Input: part model. Units: mm. Frame: model coordinates. A direction names the side the tool comes from. Coordinates: 2 decimals unless noted, no trailing zeros. Loops run counter-clockwise (first coordinate to the right, second up) from the corner with the lowest first, then second, coordinate; pieces in that order, holes last.
(1) Section B-B, the plane y = 36. Return loops of the section in (x, z).
(2) Section A-A, the plane x = 65. Return loops of the section in (y, z), then the cut area to 3 significant figures.
(3) Line query: L1, parallel to Y at x = 65, z = 6.25; L2, parallel to X at y = 36, z = 5; L3, parallel to Z at x = 35.5, y = 26. Output: solid intervals per line, ascending.
(4) Section D-D, the plane y = 20.5. Return loops of the section in (x, z), then the cut area to 3 significant figures.
(5) Contact query for flat-ended pins moving along their axis: P1, Ø1, axis at x = 39, z = 14, coming from the +Y side; P2, Ø1.6, axis at y = 5.5, z = 14.5, coming from the -X side. Output: stop coordinate, or through.
(6) Set-up query: faces 4 (the face through (49, 7, 14)), 5 (the face through (19, 7, 14)), 6 (the face through (34, 14, 14)). Return all of +Z, -Z, +X, -X, +Y, -Y with unobstructed straight access to the full face (end or side cutting, diameter ignored); none if empty.
(7) Mould query, pull axis Y, two halves, no side actions, for faces 1 (the face through (67.4, 0.57, 6.59)), 2 (the face through (3.325, 37.464, 6.409)), 3 (the face through (34, 20, 0)). Classes: released by +Y, released by -Y, zero draft, split by the parting line, or undercut.
(8) Section C-C, the plane x = 32.5. Return loops of the section in (y, z), then the cut area to 3 significant figures.
```python
from build123d import *

# Parameters (mm, degrees)
CROQUIS1_W              = 68
CROQUIS1_H              = 39
CROQUIS1_R              = 1.5
SALIENTE_EXTRUIR1_DEPTH = 13
REDONDEO1_R             = 2
CROQUIS2_W              = 30
CROQUIS2_H              = 14
SALIENTE_EXTRUIR2_DEPTH = 2


with BuildPart() as part:
    # Croquis1 → Saliente-Extruir1 (new body)
    with BuildSketch(Plane.XY):
        with Locations((34, 19.5)):
            Rectangle(CROQUIS1_W, CROQUIS1_H)
        with Locations(Location((3, 36, 0), (0, 0, 180))):
            Circle(CROQUIS1_R, mode=Mode.SUBTRACT)
        with Locations(Location((3, 3, 0), (0, 0, 180))):
            Circle(CROQUIS1_R, mode=Mode.SUBTRACT)
        with Locations(Location((65, 36, 0), (0, 0, 180))):
            Circle(CROQUIS1_R, mode=Mode.SUBTRACT)
        with Locations(Location((65, 3, 0), (0, 0, 180))):
            Circle(CROQUIS1_R, mode=Mode.SUBTRACT)
    extrude(amount=SALIENTE_EXTRUIR1_DEPTH)

    # Redondeo1
    redondeo1_edges = [part.edges().sort_by_distance(p)[0] for p in [
        (0, 39, 6.5),
        (68, 39, 6.5),
        (68, 0, 6.5),
        (0, 0, 6.5),
    ]]
    fillet(redondeo1_edges, radius=REDONDEO1_R)

    # Croquis2 → Saliente-Extruir2 (add)
    with BuildSketch(Plane.XY.offset(13)):
        with Locations((34, 7)):
            Rectangle(CROQUIS2_W, CROQUIS2_H)
    extrude(amount=SALIENTE_EXTRUIR2_DEPTH)


solid = part.part
```
Report:
1. outline: (0, 0) - (1.5, 0) - (1.5, 13) - (0, 13) - close; (4.5, 0) - (63.5, 0) - (63.5, 13) - (4.5, 13) - close; (66.5, 0) - (68, 0) - (68, 13) - (66.5, 13) - close
2. outline: (0, 0) - (1.5, 0) - (1.5, 13) - (0, 13) - close; (4.5, 0) - (34.5, 0) - (34.5, 13) - (4.5, 13) - close; (37.5, 0) - (39, 0) - (39, 13) - (37.5, 13) - close
2. area: 429 mm2
3. L1: y = 0 to 1.5, 4.5 to 34.5, 37.5 to 39
3. L2: x = 0 to 1.5, 4.5 to 63.5, 66.5 to 68
3. L3: z = 0 to 13
4. outline: (0, 0) - (68, 0) - (68, 13) - (0, 13) - close
4. area: 884 mm2
5. P1: stops at y = 14
5. P2: stops at x = 19
6. face 4: +Z, +X, +Y, -Y
6. face 5: +Z, -X, +Y, -Y
6. face 6: +Z, +X, -X, +Y
7. face 1: released by -Y
7. face 2: undercut
7. face 3: zero draft
8. outline: (0, 0) - (39, 0) - (39, 13) - (14, 13) - (14, 15) - (0, 15) - close
8. area: 535 mm2
